Design review of the part built by this model. Coordinates are the model's own, in mm. Round coordinates to 2 decimals unless told otherwise and drop trailing zeros. Write each loop counter-clockwise with the first axis right and the second up, starting at its lowest first coordinate (ties: lowest second). Pieces come first, ordered by that corner, then holes. Notation, with made-up numbers: (-19.5, 83) -> (29.5, 83) arc R30 ccw to (29.5, 117) -> close; hole circle Ø1 at (65, -3.75). An arc over 180 degrees is marked (long way). One line per question, with ' | ' between items. Start each with the question number.
1) Insertion check: pin 1 Ø12 at (x, y) = (2, 14) entering from -Z; pin 2 Ø8 at (x, z) = (-5, 9.5) entering from +Y; pin 3 Ø2.5 at (x, y) = (15.56, 15.56) entering from -Z; pin 4 Ø1.5 at (y, z) = (15.5, 8) entering from +X. Each pin has a flat end and moves straight along its axis. Give the tip position at first contact, or say it passes through.
2) Consider section D-D (x = 13). Give the boundary of the cut face in (y, z).
3) Consider section C-C (z = 14.5). Give the boundary of the cut face in (x, y).
4) For probe 1 along Y at (x, z) = (0, 4); probe 2 along Y at (x, z) = (-14.5, 8.5); probe 3 along X at (y, z) = (0.5, 1.25), list the stretches that pass through material, from the lowest coordinate up.
5) Consider section A-A (y = 0). Give the boundary of the cut face in (x, z), then the cut area to 3 significant figures.
```python
from build123d import *

# Parameters (mm, degrees)
SKETCH1_R           = 30
SKETCH1_R_2         = 1.5
BOSS_EXTRUDE1_DEPTH = 16
SKETCH2_R           = 1.6
CUT_EXTRUDE2_DEPTH  = 17


with BuildPart() as part:
    # Sketch1 → Boss-Extrude1 (new body)
    with BuildSketch(Plane.XY):
        Circle(SKETCH1_R)
        Circle(SKETCH1_R_2, mode=Mode.SUBTRACT)
    extrude(amount=BOSS_EXTRUDE1_DEPTH)

    # Sketch2 → Cut-Extrude2 (cut)
    with BuildSketch(Plane.XY):
        with Locations((15.556349186, 15.556349186)):
            Circle(SKETCH2_R)
        with Locations((-15.556349186, 15.556349186)):
            Circle(SKETCH2_R)
        with Locations((-15.556349186, -15.556349186)):
            Circle(SKETCH2_R)
        with Locations((15.556349186, -15.556349186)):
            Circle(SKETCH2_R)
    extrude(amount=CUT_EXTRUDE2_DEPTH, mode=Mode.SUBTRACT)


solid = part.part
```
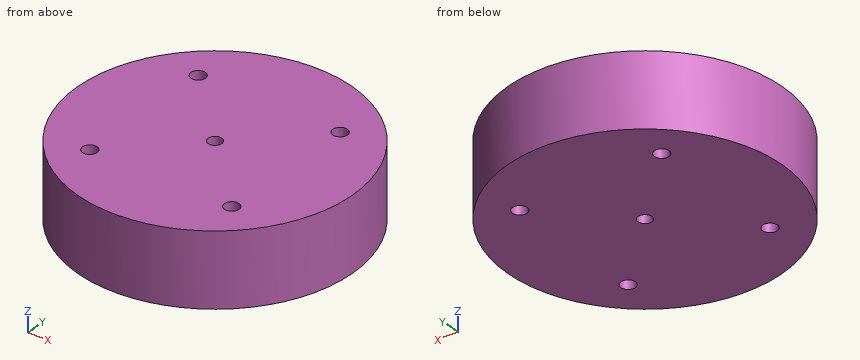
From the geometry:
1) pin 1: stops at z = 0 | pin 2: stops at y = 29.98 | pin 3: passes through | pin 4: stops at x = 26.12
2) outline: (-27.04, 0) -> (27.04, 0) -> (27.04, 16) -> (-27.04, 16) -> close
3) outline: circle Ø60 at (0, 0); hole circle Ø3.2 at (-15.56, -15.56); hole circle Ø3.2 at (-15.56, 15.56); hole circle Ø3 at (0, 0); hole circle Ø3.2 at (15.56, -15.56); hole circle Ø3.2 at (15.56, 15.56)
4) probe 1: y = -30 to -1.5, 1.5 to 30 | probe 2: y = -26.26 to -16.76, -14.35 to 14.35, 16.76 to 26.26 | probe 3: x = -30 to -1.41, 1.41 to 30
5) outline: (-30, 0) -> (-1.5, 0) -> (-1.5, 16) -> (-30, 16) -> close; (1.5, 0) -> (30, 0) -> (30, 16) -> (1.5, 16) -> close | area: 912 mm2
